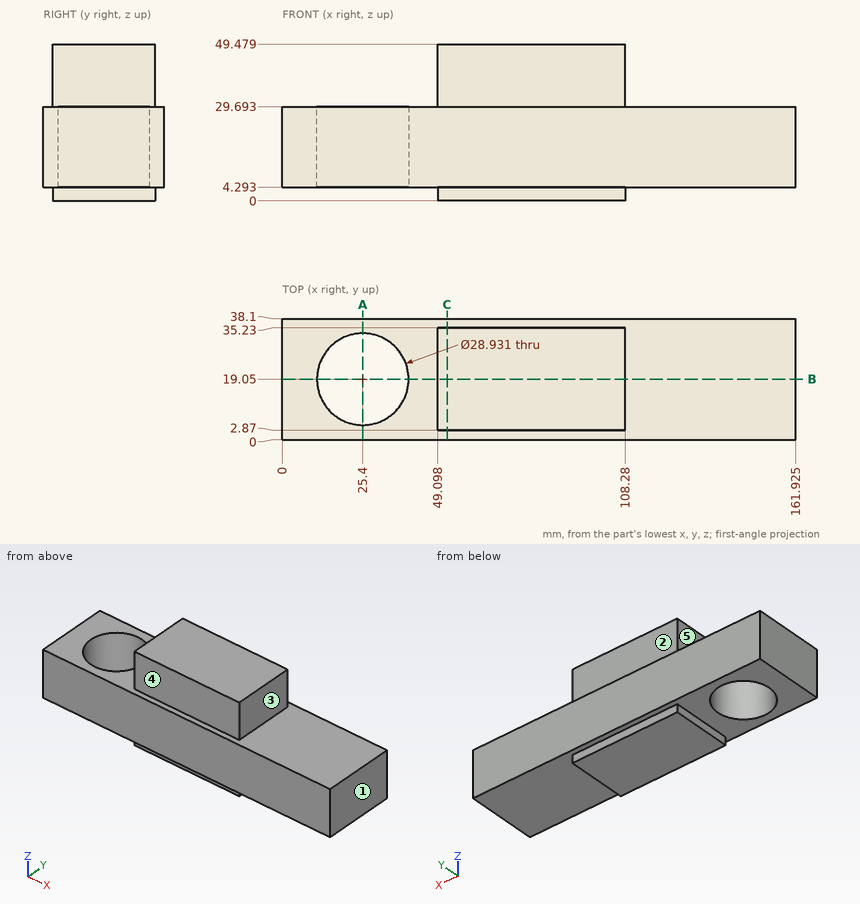
Geometry: see drawing. Coordinates: mm, zero at the bounding-box minimum. A direction names the side the tool comes from. Round coordinates to 2 decimals unless told otherwise and drop trailing zeros. Write each loop counter-clockwise with the first axis right and the second up, starting at its lowest first coordinate (ties: lowest second). Pieces come first, ordered by that corner, then holes. Notation, with made-up numbers: (38.25, -23) - (49.25, -23) arc R26 cw to (49.25, -4) - close; hole circle Ø11 at (26, 49.5). An arc over 180 degrees is marked (long way). Use CSV: the item, a comma, the result in double quotes. Start each with the question number.
(1) First-contact query: pin 1 Ø2 at (y, z) = (9, 32.5) entering from +X; pin 2 Ø16 at (y, z) = (19, 44.5) entering from -X; pin 3 Ø1.3 at (x, z) = (87.5, 1) entering from -Y. Flat tips, straight axial feed; report the tip coordinate or a pass-through.
(2) Cut plane B-B, the plane y = 19.05. Return loops of the section in (x, z) (1 decimal).
(3) Cut plane C-C, the plane x = 52. Return loops of the section in (y, z), and give its area (3 significant figures).
(4) Set-up query: the marked faces 1, 2, 3, 4 and 5. Return all of +Z, -Z, +X, -X, +Y, -Y with unobstructed straight access to the full face (end or side cutting, diameter ignored); none if empty.
(5) Material intervals for probe 1 along X at (y, z) = (19, 24) (1 decimal); probe 2 along Y at (x, z) = (25, 12); probe 3 along Z at (x, y) = (49, 27.5), sorted ascending. Write a range as [from, to].
(6) Cut plane A-A, the plane x = 25.4. Return loops of the section in (y, z) (1 decimal).
Geometry says:
1,pin 1,"x = 108.28"
1,pin 2,"x = 49.1"
1,pin 3,"y = 2.87"
2,outline,"(0, 4.3) - (10.9, 4.3) - (10.9, 29.7) - (0, 29.7) - close; (39.9, 4.3) - (49.1, 4.3) - (49.1, 0) - (108.3, 0) - (108.3, 4.3) - (161.9, 4.3) - (161.9, 29.7) - (108.3, 29.7) - (108.3, 49.5) - (49.1, 49.5) - (49.1, 29.7) - (39.9, 29.7) - close"
3,outline,"(0, 4.29) - (2.87, 4.29) - (2.87, 0) - (35.23, 0) - (35.23, 4.29) - (38.1, 4.29) - (38.1, 29.69) - (35.23, 29.69) - (35.23, 49.48) - (2.87, 49.48) - (2.87, 29.69) - (0, 29.69) - close"
3,area,"1,750 mm²"
4,face 1,"+Z, -Z, +X, +Y, -Y"
4,face 2,"+Z, +X, -X, +Y"
4,face 3,"+Z, +X, +Y, -Y"
4,face 4,"+Z, +X, -X, -Y"
4,face 5,"+Z, -X, +Y, -Y"
5,probe 1,"[0, 10.9], [39.9, 161.9]"
5,probe 2,"[0, 4.59], [33.51, 38.1]"
5,probe 3,"[4.29, 29.69]"
6,outline,"(0, 4.3) - (4.6, 4.3) - (4.6, 29.7) - (0, 29.7) - close; (33.5, 4.3) - (38.1, 4.3) - (38.1, 29.7) - (33.5, 29.7) - close"
